Build history of the part. All positions in model axes, mm. Face numbers are marked on the shaded views. A direction names the side the tool comes from. Round coordinates to 2 decimals unless told otherwise and drop trailing zeros. Answer as a JSON object with one key per item and string values. Group by question number.
Item 1: Slice it at A-A, the plane x = 10.25. Give the number of separate pieces and of enclosed holes in the cut face, then the cut area to 3 significant figures.
Item 2: Flat gauge pins, fed straight in: pin 1 (12 mm diameter, centred on y = 11, z = 6, fed in from -X); pin 2 (6 mm diameter, centred on x = 15.5, z = -23, fed in from +Y); pin 3 (0.6 mm diameter, centred on x = 18.5, y = 0, fed in from -Z). Where does each tip first touch, or does it go through?
Item 3: Which spindle directions (+Z, -Z, +X, -X, +Y, -Y) get a long thin tool onto all of the face, cutting with end or side? Do the marked faces 1, 2 and 3. Say none if no direction does.
Item 4: Probe line 1 (Y direction, x = 1.55, z = 0); line 2 (Y direction, x = 19.4, z = 0); line 3 (Y direction, x = 3.25, z = 21.5). List the from-to ranges inside material, lowest first. Write a range as from..to.
from build123d import *

# Parameters (mm, degrees)
SKETCH1_R           = 50
BOSS_EXTRUDE1_DEPTH = 20
SKETCH2_R           = 40
CUT_EXTRUDE1_DEPTH  = 2
CUT_EXTRUDE2_DEPTH  = 73.965745388
CIRPATTERN1_COUNT   = 13
FILLET1_R           = 5
BOSS_EXTRUDE2_DEPTH = 2


with BuildPart() as part:
    # Sketch1 → Boss-Extrude1 (new body)
    with BuildSketch(Plane(origin=(0, 0, 0), x_dir=(0, 0, -1), z_dir=(1, 0, 0))):
        Circle(SKETCH1_R)
    extrude(amount=BOSS_EXTRUDE1_DEPTH)

    # Sketch2 → Cut-Extrude1 (cut)
    with BuildSketch(Plane.ZY):
        Circle(SKETCH2_R)
    cut_extrude1 = extrude(amount=-CUT_EXTRUDE1_DEPTH, mode=Mode.SUBTRACT)

    # Mirror1: Cut-Extrude1 across plane
    add(cut_extrude1.mirror(Plane(origin=(10, 0, 0), x_dir=(0, 0, 1), z_dir=(1, 0, 0))), mode=Mode.SUBTRACT)

    # Sketch3 → Cut-Extrude2 (cut, through all)
    with BuildSketch(Plane.ZY.offset(-2)):
        with BuildLine():
            Line((0, 38), (0, 5))
            ThreePointArc((0, 5), (0.327015646, 4.989294616), (0.652630961, 4.957224307))
            Line((0.652630961, 4.957224307), (4.959995304, 37.674904732))
            ThreePointArc((4.959995304, 37.674904732), (2.485318911, 37.918639083), (0, 38))
        make_face()
        with BuildLine():
            ThreePointArc((-0.652630961, 4.957224307), (-0.327015646, 4.989294616), (0, 5))
            Line((0, 5), (0, 38))
            ThreePointArc((0, 38), (-2.485318911, 37.918639083), (-4.959995304, 37.674904732))
            Line((-4.959995304, 37.674904732), (-0.652630961, 4.957224307))
        make_face()
    cut_extrude2 = extrude(amount=-CUT_EXTRUDE2_DEPTH, mode=Mode.SUBTRACT)

    # CirPattern1: Cut-Extrude2 ×13 about axis
    cirpattern1_axis = Axis((0, 0, 0), (1, 0, 0))
    for i in range(1, CIRPATTERN1_COUNT):
        add(cut_extrude2.rotate(cirpattern1_axis, i * 360 / CIRPATTERN1_COUNT), mode=Mode.SUBTRACT)

    # Fillet1
    fillet1_edges = [part.edges().sort_by_distance(p)[0] for p in [
        (0, 0, 50),
        (20, 0, 50),
    ]]
    fillet(fillet1_edges, radius=FILLET1_R)

    # Sketch4 → Boss-Extrude2 (add)
    with BuildSketch(Plane.ZY.offset(-2)):
        Polygon((0, -2.886751346), (2.5, -1.443375673), (2.5, 1.443375673), (0, 2.886751346), (-2.5, 1.443375673), (-2.5, -1.443375673), align=None)
    boss_extrude2 = extrude(amount=BOSS_EXTRUDE2_DEPTH)

    # Mirror2: Boss-Extrude2 across plane
    add(boss_extrude2.mirror(Plane(origin=(10, 0, 0), x_dir=(0, 0, 1), z_dir=(1, 0, 0))))


solid = part.part
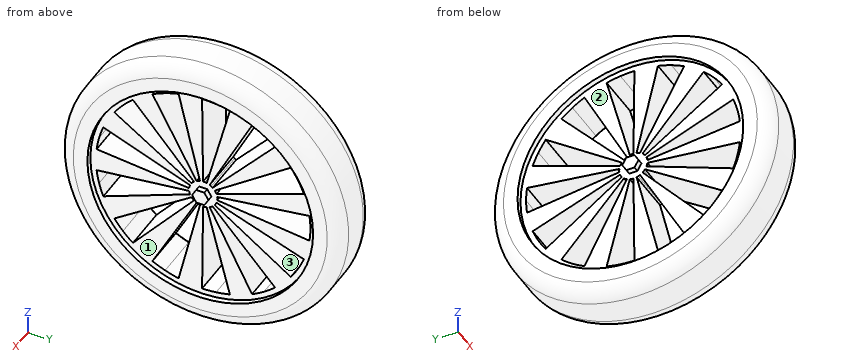
Geometry says:
{
 "1": {"separate pieces": "1", "enclosed holes": "13", "area": "5,440 mm^2"},
 "2": {"pin 1": "stops at x = 2", "pin 2": "stops at y = 45.81", "pin 3": "stops at z = -48.84"},
 "3": {"face 1": "+X", "face 2": "-X", "face 3": "+X, -X"},
 "4": {"line 1": "y = -48.62..-40, -2.89..2.89, 40..48.62", "line 2": "y = -47.37..-40, -2.89..2.89, 40..47.37", "line 3": "y = -44.79..-31.33, -18.66..-11.56, -5.07..-0.22, 5.53..11.01, 19.44..30.49, 31.33..44.79"}
}
